Read the model definition and answer for the solid it produces. Units are mm, in the model's axes. Round coordinates to 2 decimals unless told otherwise and drop trailing zeros. Use one line per item in the form item = value. Start each with the question number.
from build123d import *

# Parameters (mm, degrees)
SKETCH_1_R              = 2.1
SKETCH_1_R_2            = 3.4
F_30XS6_30X60S6_1_DEPTH = 600


with BuildPart() as part:
    # 草图1 → 30xs6 30X60S6(1) (new body)
    with BuildSketch(Plane.ZY):
        with BuildLine():
            Line((-13, -30), (-4.3, -30))
            ThreePointArc((-4.3, -30), (-4.087867966, -29.912132034), (-4, -29.7))
            Line((-4, -29.7), (-4, -28))
            Line((-4, -28), (-8.249999995, -28))
            Line((-8.249999995, -28), (-8.249999995, -24.664213567))
            Line((-8.249999995, -24.664213567), (-4.585786428, -21))
            Line((-4.585786428, -21), (-0.519615237, -21))
            Line((-0.519615237, -21), (5e-09, -20.7))
            Line((5e-09, -20.7), (0.519615247, -21))
            Line((0.519615247, -21), (4.585786438, -21))
            Line((4.585786438, -21), (8.250000005, -24.664213567))
            Line((8.250000005, -24.664213567), (8.250000005, -28))
            Line((8.250000005, -28), (4, -28))
            Line((4, -28), (4, -29.7))
            ThreePointArc((4, -29.7), (4.087867966, -29.912132034), (4.3, -30))
            Line((4.3, -30), (13, -30))
            ThreePointArc((13, -30), (14.414213562, -29.414213562), (15, -28))
            Line((15, -28), (15, -19.3000023))
            ThreePointArc((15, -19.3000023), (14.912132034, -19.087870266), (14.7, -19.0000023))
            Line((14.7, -19.0000023), (13.000000005, -19.0000023))
            Line((13.000000005, -19.0000023), (13.000000005, -23.250000005))
            Line((13.000000005, -23.250000005), (9.664213567, -23.250000005))
            Line((9.664213567, -23.250000005), (6.000000005, -19.585786443))
            Line((6.000000005, -19.585786443), (6.000000005, -15.519615247))
            Line((6.000000005, -15.519615247), (5.700000005, -15.000000005))
            Line((5.700000005, -15.000000005), (6.000000005, -14.480384763))
            Line((6.000000005, -14.480384763), (6.000000005, -10.414213567))
            Line((6.000000005, -10.414213567), (9.664213567, -6.750000005))
            Line((9.664213567, -6.750000005), (13.000000005, -6.750000005))
            Line((13.000000005, -6.750000005), (13.000000005, -11.0000023))
            Line((13.000000005, -11.0000023), (14.7, -11.0000023))
            ThreePointArc((14.7, -11.0000023), (14.912132034, -10.912134335), (15, -10.7000023))
            Line((15, -10.7000023), (15, 10.7000023))
            ThreePointArc((15, 10.7000023), (14.912132034, 10.912134335), (14.7, 11.0000023))
            Line((14.7, 11.0000023), (13.000000005, 11.0000023))
            Line((13.000000005, 11.0000023), (13.000000005, 6.749999995))
            Line((13.000000005, 6.749999995), (9.664213567, 6.749999995))
            Line((9.664213567, 6.749999995), (6.000000005, 10.414213557))
            Line((6.000000005, 10.414213557), (6.000000005, 14.480384753))
            Line((6.000000005, 14.480384753), (5.700000005, 14.999999995))
            Line((5.700000005, 14.999999995), (6.000000005, 15.519615237))
            Line((6.000000005, 15.519615237), (6.000000005, 19.585786433))
            Line((6.000000005, 19.585786433), (9.664213567, 23.249999995))
            Line((9.664213567, 23.249999995), (13.000000005, 23.249999995))
            Line((13.000000005, 23.249999995), (13.000000005, 19.0000023))
            Line((13.000000005, 19.0000023), (14.7, 19.0000023))
            ThreePointArc((14.7, 19.0000023), (14.912132034, 19.087870266), (15, 19.3000023))
            Line((15, 19.3000023), (15, 28))
            ThreePointArc((15, 28), (14.414213562, 29.414213562), (13, 30))
            Line((13, 30), (4.3, 30))
            ThreePointArc((4.3, 30), (4.087867966, 29.912132034), (4, 29.7))
            Line((4, 29.7), (4, 28))
            Line((4, 28), (8.250000005, 28))
            Line((8.250000005, 28), (8.250000005, 24.664213557))
            Line((8.250000005, 24.664213557), (4.585786448, 21))
            Line((4.585786448, 21), (0.519615247, 21))
            Line((0.519615247, 21), (5e-09, 20.7))
            Line((5e-09, 20.7), (-0.519615237, 21))
            Line((-0.519615237, 21), (-4.585786438, 21))
            Line((-4.585786438, 21), (-8.249999995, 24.664213557))
            Line((-8.249999995, 24.664213557), (-8.249999995, 28))
            Line((-8.249999995, 28), (-4, 28))
            Line((-4, 28), (-4, 29.7))
            ThreePointArc((-4, 29.7), (-4.087867966, 29.912132034), (-4.3, 30))
            Line((-4.3, 30), (-13, 30))
            ThreePointArc((-13, 30), (-14.414213562, 29.414213562), (-15, 28))
            Line((-15, 28), (-15, 19.3000023))
            ThreePointArc((-15, 19.3000023), (-14.912132034, 19.087870266), (-14.7, 19.0000023))
            Line((-14.7, 19.0000023), (-12.999999995, 19.0000023))
            Line((-12.999999995, 19.0000023), (-12.999999995, 23.249999995))
            Line((-12.999999995, 23.249999995), (-9.664213557, 23.249999995))
            Line((-9.664213557, 23.249999995), (-5.999999995, 19.585786433))
            Line((-5.999999995, 19.585786433), (-5.999999995, 15.519615237))
            Line((-5.999999995, 15.519615237), (-5.699999995, 14.999999995))
            Line((-5.699999995, 14.999999995), (-5.999999995, 14.480384753))
            Line((-5.999999995, 14.480384753), (-5.999999995, 10.414213557))
            Line((-5.999999995, 10.414213557), (-9.664213557, 6.749999995))
            Line((-9.664213557, 6.749999995), (-12.999999995, 6.749999995))
            Line((-12.999999995, 6.749999995), (-12.999999995, 11.0000023))
            Line((-12.999999995, 11.0000023), (-14.7, 11.0000023))
            ThreePointArc((-14.7, 11.0000023), (-14.912132034, 10.912134335), (-15, 10.7000023))
            Line((-15, 10.7000023), (-15, -10.7000023))
            ThreePointArc((-15, -10.7000023), (-14.912132034, -10.912134335), (-14.7, -11.0000023))
            Line((-14.7, -11.0000023), (-12.999999995, -11.0000023))
            Line((-12.999999995, -11.0000023), (-12.999999995, -6.750000005))
            Line((-12.999999995, -6.750000005), (-9.664213557, -6.750000005))
            Line((-9.664213557, -6.750000005), (-5.999999995, -10.414213567))
            Line((-5.999999995, -10.414213567), (-5.999999995, -14.480384763))
            Line((-5.999999995, -14.480384763), (-5.699999995, -15.000000005))
            Line((-5.699999995, -15.000000005), (-5.999999995, -15.519615247))
            Line((-5.999999995, -15.519615247), (-5.999999995, -19.585786443))
            Line((-5.999999995, -19.585786443), (-9.664213557, -23.250000005))
            Line((-9.664213557, -23.250000005), (-12.999999995, -23.250000005))
            Line((-12.999999995, -23.250000005), (-12.999999995, -19.0000023))
            Line((-12.999999995, -19.0000023), (-14.7, -19.0000023))
            ThreePointArc((-14.7, -19.0000023), (-14.912132034, -19.087870266), (-15, -19.3000023))
            Line((-15, -19.3000023), (-15, -28))
            ThreePointArc((-15, -28), (-14.414213562, -29.414213562), (-13, -30))
        make_face()
        with Locations((11.625000005, 26.624999995)):
            Circle(SKETCH_1_R, mode=Mode.SUBTRACT)
        with Locations((11.625000005, -26.625000005)):
            Circle(SKETCH_1_R, mode=Mode.SUBTRACT)
        with Locations((4.55e-07, -15.00000049)):
            Circle(SKETCH_1_R_2, mode=Mode.SUBTRACT)
        with Locations((4.55e-07, 15.0000023)):
            Circle(SKETCH_1_R_2, mode=Mode.SUBTRACT)
        with Locations((-11.624999995, 26.624999995)):
            Circle(SKETCH_1_R, mode=Mode.SUBTRACT)
        with Locations((-11.624999995, -26.625000005)):
            Circle(SKETCH_1_R, mode=Mode.SUBTRACT)
        with BuildLine():
            Line((-12.999999995, 3.749999995), (-12.999999995, -3.750000005))
            ThreePointArc((-12.999999995, -3.750000005), (-12.707106776, -4.457106786), (-11.999999995, -4.750000005))
            Line((-11.999999995, -4.750000005), (-8.835786433, -4.750000005))
            Line((-8.835786433, -4.750000005), (-3.651790591, -9.933995846))
            ThreePointArc((-3.651790591, -9.933995846), (-3.470778838, -10.020245326), (-3.275865231, -9.973203714))
            ThreePointArc((-3.275865231, -9.973203714), (1.45e-07, -9.000002005), (3.275865622, -9.973203376))
            ThreePointArc((3.275865622, -9.973203376), (3.470779219, -10.02024497), (3.651790956, -9.933995491))
            Line((3.651790956, -9.933995491), (8.835786443, -4.750000005))
            Line((8.835786443, -4.750000005), (12.000000005, -4.750000005))
            ThreePointArc((12.000000005, -4.750000005), (12.707106786, -4.457106786), (13.000000005, -3.750000005))
            Line((13.000000005, -3.750000005), (13.000000005, 3.749999995))
            ThreePointArc((13.000000005, 3.749999995), (12.707106786, 4.457106776), (12.000000005, 4.749999995))
            Line((12.000000005, 4.749999995), (8.835786443, 4.749999995))
            Line((8.835786443, 4.749999995), (3.6517913, 9.933995138))
            ThreePointArc((3.6517913, 9.933995138), (3.470779584, 10.020244614), (3.275866001, 9.973203046))
            ThreePointArc((3.275866001, 9.973203046), (1.45e-07, 9.000001815), (-3.27586561, 9.973203384))
            ThreePointArc((-3.27586561, 9.973203384), (-3.470779203, 10.020244971), (-3.651790935, 9.933995493))
            Line((-3.651790935, 9.933995493), (-8.835786433, 4.749999995))
            Line((-8.835786433, 4.749999995), (-11.999999995, 4.749999995))
            ThreePointArc((-11.999999995, 4.749999995), (-12.707106776, 4.457106776), (-12.999999995, 3.749999995))
        make_face(mode=Mode.SUBTRACT)
    extrude(amount=F_30XS6_30X60S6_1_DEPTH)


solid = part.part
Item 1: Given P1, Ø3.5, axis at x = -158.5, z = -2, coming from the +Y side; P2, Ø0.5, axis at x = -347.5, z = -14, coming from the -Y side; P3, Ø2.5, axis at y = 26.625, z = -11.625, coming from the -X side; P4, Ø6, axis at x = -387.5, y = -15, coming from the +Z side, each flat-ended and moving along its own axis, determine where each tip first touches the part or whether it passes through.
Item 2: Section A-A (x = -40) is taken. Give the number of separate pieces and of enclosed holes in the cut face, and give its area (3 significant figures).
Item 3: Find the intervals of material crossed by L1, parallel to Y at x = -171.5, z = 11; L2, parallel to Z at x = -126, y = -26.5; L3, parallel to Y at x = -375, z = -2, in increasing order. Write a range as [from, to].
The answers:
q1.P1 = 21
q1.P2 = -29.85
q1.P3 = through
q1.P4 = 6
q2.separate_pieces = 1
q2.enclosed_holes = 7
q2.area = 591 mm²
q3.L1 = [-30, -28.63], [-24.62, -23.25], [-6.75, -4.75], [4.75, 6.75], [23.25, 24.62], [28.63, 30]
q3.L2 = [-15, -13.72], [-9.53, -8.25], [8.25, 9.53], [13.72, 15]
q3.L3 = [-21, -17.75], [-12.25, -9.34], [9.34, 12.25], [17.75, 21]
